Autodesk Inventor part; units mm, degrees
ref_plane "YZ Plane" through (0, 0, 0) normal (1, 0, 0) x (0, 1, 0)
ref_plane "XZ Plane" through (0, 0, 0) normal (0, 1, 0) x (-1, 0, 0)
ref_plane "XY Plane" through (0, 0, 0) normal (0, 0, 1) x (1, 0, 0)
sketch "Sketch1" plane through (0, 0, 0) normal (0, 0, 1) x (1, 0, 0)
  line L0 (-150, 125) -> (150, 125)
  line L1 (150, 125) -> (150, -125)
  line L2 (150, -125) -> (-150, -125)
  line L3 (-150, -125) -> (-150, 125)
  point P0 (0, 0)
  point P1 (0, 125)
  point P2 (150, 0)
  dimension "d0" = 300
  dimension "d1" = 250
extrude "Extrusion1" add sketch "Sketch1" along normal blind 39.37
sketch "Sketch2" plane through (0, 0, 39.37) normal (0, 0, 1) x (1, 0, 0)
  line L0 (-150, 125) -> (-150, -125)
  line L1 (150, 125) -> (-150, 125) construction
  line L2 (0, 125) -> (0, -125) construction
  line L3 (-150, -125) -> (150, -125) construction
  point P0 (0, 0)
  point P1 (-120, 0)
  point P2 (120, 0)
  dimension "d4" = 30
hole "Hole1" at (-120, 0, 39.37) at (120, 0, 39.37) direction (0, 0, -1) diameter 10 end through all
hole "Hole2" at (-120, 0, 39.37) at (120, 0, 39.37) direction (0, 0, -1) diameter 20 depth 10 tip angle 118 countersink diameter 25 countersink angle 82
properties part number "TablaInferior"
Read the model definition and answer for the solid it produces. Units are mm, in the model's axes. A direction names the side the tool comes from. Coordinates: 2 decimals unless noted, no trailing zeros. Order: outer loops, then holes, each group sorted by start corner. A loop starts at its lowest first (then second) coordinate and runs counter-clockwise, first axis right, second up. Notation, with made-up numbers: (-14, 27) - (37, 27) arc R24 cw to (37, 60) - close; hole circle Ø1 at (69.25, 68). An arc over 180 degrees is marked (long way). Use one line per item in the form item = value.
(1) For a pull along X with two mould halves and no side action, classify faces 3 (the face through (-2, 125, 19)), 4 (the face through (-150, -2, 19)), 5 (the face through (150, 2, 19)), 6 (the face through (-109.93, 1.322, 36.674)) as pulls with the +X half, pulls with the -X half, needs draft (parallel to the pull), parting line crosses it, or undercut.
Computed values:
face_3 = needs draft
face_4 = pulls with the -X half
face_5 = pulls with the +X half
face_6 = undercut
(2) Section A-A, the plane y = 0 is taken. Give the vertices of the cut face in (x, z).
Computed values:
outline = (-150, 0) - (-125, 0) - (-125, 26.37) - (-130, 29.37) - (-130, 36.49) - (-132.5, 39.37) - (-150, 39.37) - close; (-115, 0) - (115, 0) - (115, 26.37) - (110, 29.37) - (110, 36.49) - (107.5, 39.37) - (-107.5, 39.37) - (-110, 36.49) - (-110, 29.37) - (-115, 26.37) - close; (125, 0) - (150, 0) - (150, 39.37) - (132.5, 39.37) - (130, 36.49) - (130, 29.37) - (125, 26.37) - close
(3) Which of the six approach directions +Z, -Z, +X, -X, +Y, -Y give full straight-line access (tool end or side, diameter ignored) to faces 1 (the face through (2, -125, 19)), 2 (the face through (110.085, 1.302, 32.882))?
Computed values:
face_1 = +Z, -Z, +X, -X, -Y
face_2 = +Z
(4) Given pin 1 Ø9 at (x, y) = (-120, 0) entering from -Z, flat-ended and moving along its own axis, determine where the tip first touches the part or whether it passes through.
Computed values:
pin_1 = through
(5) Straight lines are drawn through the part: L1, parallel to X at y = 0, z = 5; L2, parallel to X at y = 0, z = 32; L3, parallel to Y at x = -120, z = 17. For each, find the intervals that lie inside material, in ascending order.
Computed values:
L1 = -150 to -125, -115 to 115, 125 to 150
L2 = -150 to -130, -110 to 110, 130 to 150
L3 = -125 to -5, 5 to 125
(6) Section B-B, the plane x = -120 is taken. Give the vertices of the cut face in (y, z), then the cut area to 3 significant figures.
Computed values:
outline = (-125, 0) - (-5, 0) - (-5, 26.37) - (-10, 29.37) - (-10, 36.49) - (-12.5, 39.37) - (-125, 39.37) - close; (5, 0) - (125, 0) - (125, 39.37) - (12.5, 39.37) - (10, 36.49) - (10, 29.37) - (5, 26.37) - close
area = 9,330 mm²
